Check sheet for the drawn part. Datum: minimum x, y, z corner. Units: mm. Coordinates: 2 decimals unless noted, no trailing zeros. Order: outer loops, then holes, each group sorted by start corner. A loop starts at its lowest first (then second) coordinate and runs counter-clockwise, first axis right, second up. Notation, with made-up numbers: M -3,8.25 L 38,8.25 A19 cw 38,25.25 Z; hole C 16.25,38 d3. An arc over 180 degrees is marked long. Return JSON: item names as keys, results as strings. Group by question number.
Q1. Thickness scan on probe 1 along Z at (x, y) = (35, 7.5); probe 2 along X at (y, z) = (4.5, 35); probe 3 along Z at (x, y) = (18, 3.75). Record the ranges inside material, lowest first.
Q2. Section check A-A, the plane z = 78. Enter the section's corners in (x, y), then the cut area to 3 significant figures.
Q3. Mould release check, pull along X, two halves, no side actions. Record for the marked faces 1, 2, 3 and 4: pulls with the +X half, pulls with the -X half, needs draft (parallel to the pull), parting line crosses it, or undercut.
Q4. Section check C-C, the plane y = 3.25. Enter the section's corners in (x, z).
Q5. Section check B-B, the plane x = 35. Enter the section's corners in (y, z).
Q6. Go/stop test with flat-tipped pins: pin 1 Ø4 at (y, z) = (3, 10) entering from +X; pin 2 Ø10 at (x, z) = (31.5, 17.5) entering from -Y; pin 3 Ø3 at (x, y) = (13.5, 2) entering from -Z; pin 4 Ø1 at (y, z) = (1.5, 15.5) entering from +X. Record where each tip stops, or that it passes through.
Q7. Section check D-D, the plane x = 54. Enter the section's corners in (y, z) (3 decimals), then the cut area to 3 significant figures.
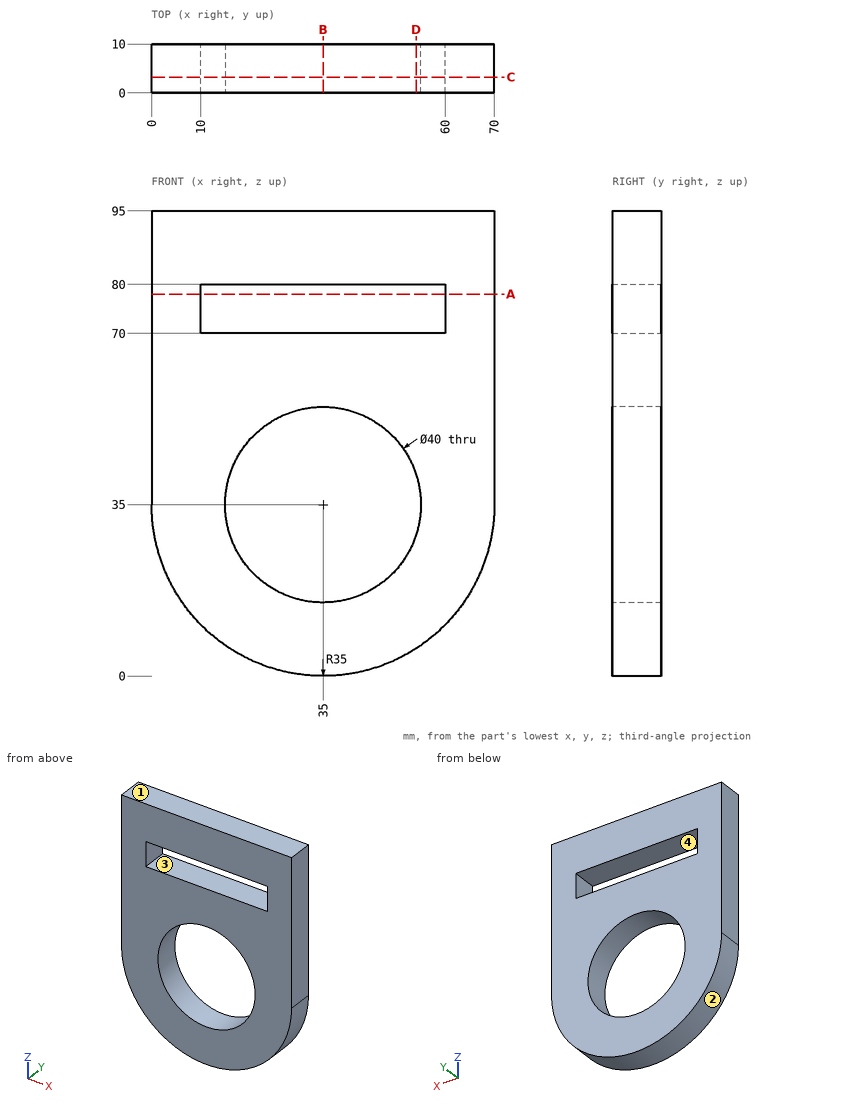
Numbers:
{
 "1": {"probe 1": "z = 0 to 15, 55 to 70, 80 to 95", "probe 2": "x = 0 to 15, 55 to 70", "probe 3": "z = 4.41 to 24.46, 45.54 to 70, 80 to 95"},
 "2": {"outline": "M 0,0 L 10,0 L 10,10 L 0,10 Z; M 60,0 L 70,0 L 70,10 L 60,10 Z", "area": "200 mm2"},
 "3": {"face 1": "needs draft", "face 2": "parting line crosses it", "face 3": "undercut", "face 4": "undercut"},
 "4": {"outline": "M 0,35 A35 ccw 70,35 L 70,95 L 0,95 Z; hole M 10,70 L 60,70 L 60,80 L 10,80 Z; hole C 35,35 d40"},
 "5": {"outline": "M 0,0 L 10,0 L 10,15 L 0,15 Z; M 0,55 L 10,55 L 10,70 L 0,70 Z; M 0,80 L 10,80 L 10,95 L 0,95 Z"},
 "6": {"pin 1": "stops at x = 61.38", "pin 2": "stops at y = 0", "pin 3": "stops at z = 6.28", "pin 4": "stops at x = 64.39"},
 "7": {"outline": "M 0,5.606 L 10,5.606 L 10,28.755 L 0,28.755 Z; M 0,41.245 L 10,41.245 L 10,70 L 0,70 Z; M 0,80 L 10,80 L 10,95 L 0,95 Z", "area": "669 mm2"}
}
